```python
from build123d import *

# Parameters (mm, degrees)
SKETCH_1_R               = 50
SKETCH_1_R_2             = 21
EXTRUDE_1_DEPTH          = 17
EXTRUDE_START            = 4
SKETCH_2_R               = 50
EXTRUDE_2_DEPTH          = 4
CUT_EXTRUDE_1_DEPTH      = 74.763134424
CUT_EXTRUDE_1_DEPTH_BACK = 74.763134424
SKETCH_3_R               = 4
SKETCH_3_R_2             = 1.55


with BuildPart() as part:
    # 草图1 → 凸台-拉伸1 (new body)
    with BuildSketch(Plane.XY):
        Circle(SKETCH_1_R)
        Circle(SKETCH_1_R_2, mode=Mode.SUBTRACT)
    extrude(amount=EXTRUDE_1_DEPTH)

    # 草图2 → 凸台-拉伸2 (add)
    with BuildSketch(Plane(origin=(0, 0, 0), x_dir=(-1, 0, 0), z_dir=(0, 0, -1)).offset(EXTRUDE_START)):
        Circle(SKETCH_2_R)
    extrude(amount=-EXTRUDE_2_DEPTH)

    # 草图3 → 切除-拉伸1 (cut, two sides: drawn at the far end of the back side and taken through both)
    with BuildSketch(Plane(origin=(0, 0, -4), x_dir=(-1, 0, 0), z_dir=(0, 0, -1)).offset(-CUT_EXTRUDE_1_DEPTH_BACK)):
        Circle(SKETCH_3_R)
        with Locations((0, 6)):
            Circle(SKETCH_3_R_2)
        with Locations((0, -6)):
            Circle(SKETCH_3_R_2)
        with Locations((-6.5, 0)):
            Circle(SKETCH_3_R_2)
        with Locations((6.5, 0)):
            Circle(SKETCH_3_R_2)
    extrude(amount=CUT_EXTRUDE_1_DEPTH + CUT_EXTRUDE_1_DEPTH_BACK, mode=Mode.SUBTRACT)


solid = part.part
```
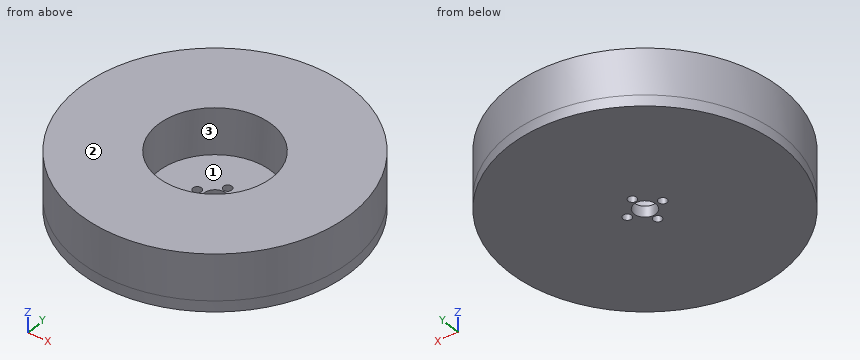
Can you work these out from the model? Positions are in its coordinate system, mm. Face numbers are marked on the shaded views. Round coordinates to 2 decimals unless told otherwise and drop trailing zeros. Order: outer loops, then holes, each group sorted by start corner. A loop starts at its lowest first (then second) coordinate and runs counter-clockwise, first axis right, second up.
(1) I'm going to push flat-ended pins straight in: pin 1 (4 mm diameter, centred on x = -6.5, y = 0, fed in from -Z); pin 2 (2 mm diameter, centred on x = -35, z = 4, fed in from -Y); pin 3 (10 mm diameter, centred on x = -38.5, z = 14.5, fed in from +Y); pin 4 (4 mm diameter, centred on x = 0, y = 6, fed in from +Z). Where does each tip first touch, or does it pass through?
Results are:
pin 1: stops at z = -4
pin 2: stops at y = -36.66
pin 3: stops at y = 37.12
pin 4: stops at z = 0
(2) If we section it at D-D (y = -12.5): Please give me the cut outline in (x, z).
Results are:
outline: (-48.41, -4) - (48.41, -4) - (48.41, 17) - (16.87, 17) - (16.87, 0) - (-16.87, 0) - (-16.87, 17) - (-48.41, 17) - close
(3) We'd pull the mould along Y, two halves only. Please class the marked faces 1, 2 and 3: +Y half, -Y half, draft (parallel to the pull), parting line (faces both ways), or undercut.
Results are:
face 1: undercut
face 2: draft
face 3: undercut
(4) If we section it at B-B (x = 0): Please give me the cut outline in (y, z), plus the area to 3 significant figures.
Results are:
outline: (-50, -4) - (-7.55, -4) - (-7.55, 0) - (-21, 0) - (-21, 17) - (-50, 17) - close; (-4.45, -4) - (-4, -4) - (-4, 0) - (-4.45, 0) - close; (4, -4) - (4.45, -4) - (4.45, 0) - (4, 0) - close; (7.55, -4) - (50, -4) - (50, 17) - (21, 17) - (21, 0) - (7.55, 0) - close
area: 1,330 mm2
(5) If we section it at A-A (y = 0): Please give me the cut outline in (x, z), plus the area to 3 significant figures.
Results are:
outline: (-50, -4) - (-8.05, -4) - (-8.05, 0) - (-21, 0) - (-21, 17) - (-50, 17) - close; (-4.95, -4) - (-4, -4) - (-4, 0) - (-4.95, 0) - close; (4, -4) - (4.95, -4) - (4.95, 0) - (4, 0) - close; (8.05, -4) - (50, -4) - (50, 17) - (21, 17) - (21, 0) - (8.05, 0) - close
area: 1,330 mm2
(6) If I drill on L1, parallel to X at y = 0, z = -1.7; L2, parallel to Y at x = 0, z = -0.9; L3, parallel to X at y = 17, z = 4, over which ranges is the centre line in solid material (lowest first)?
Results are:
L1: x = -50 to -8.05, -4.95 to -4, 4 to 4.95, 8.05 to 50
L2: y = -50 to -7.55, -4.45 to -4, 4 to 4.45, 7.55 to 50
L3: x = -47.02 to -12.33, 12.33 to 47.02
(7) If we section it at C-C (z = 3.75): Please give me the cut outline in (x, y), plus the area to 3 significant figures.
Results are:
outline: circle Ø100 at (0, 0); hole circle Ø42 at (0, 0)
area: 6,470 mm2
